Work out the finished part from the listing and answer in its coordinate system (mm). A direction names the side the tool comes from. Give positions to 0.01 mm unless a question says otherwise; leave off trailing zeros. Loops run counter-clockwise (first coordinate to the right, second up) from the corner with the lowest first, then second, coordinate; pieces in that order, holes last. Notation, with made-up numbers: M 27.5,73 L 70.5,73 A22 ccw 70.5,89 Z; hole C 10,76 d8. An arc over 180 degrees is marked long. Answer in a Markdown table with one row per item. Add a question column.
from build123d import *

# Parameters (mm, degrees)
SKETCH_1_W          = 50
SKETCH_1_H          = 15
EXTRUDE_1_DEPTH     = 18.8
SKETCH_2_W          = 46.4
SKETCH_2_H          = 15
CUT_EXTRUDE_1_DEPTH = 0.8
SKETCH_4_W          = 8.2
SKETCH_4_H          = 15
CUT_EXTRUDE_2_DEPTH = 9
SKETCH_5_W          = 8.2
SKETCH_5_H          = 1.9
CUT_EXTRUDE_3_DEPTH = 15
SKETCH_6_W          = 1.5
SKETCH_6_H          = 0.75
EXTRUDE_2_DEPTH     = 5.8
SKETCH_7_R          = 2.25
CUT_EXTRUDE_4_DEPTH = 31.004832944
CUT_EXTRUDE_START   = -30
CUT_EXTRUDE_5_DEPTH = 30


with BuildPart() as part:
    # 草图1 → 拉伸1 (new body)
    with BuildSketch(Plane(origin=(0, 0, 0), x_dir=(1, 0, 0), z_dir=(0, 1, 0))):
        Rectangle(SKETCH_1_W, SKETCH_1_H)
    extrude(amount=EXTRUDE_1_DEPTH)

    # 草图2 → 切除-拉伸1 (cut)
    with BuildSketch(Plane(origin=(0, 18.8, 0), x_dir=(-1, 0, 0), z_dir=(0, 1, 0))):
        Rectangle(SKETCH_2_W, SKETCH_2_H)
    extrude(amount=-CUT_EXTRUDE_1_DEPTH, mode=Mode.SUBTRACT)

    # 草图4 → 切除-拉伸2 (cut)
    with BuildSketch(Plane(origin=(0, 18, 0), x_dir=(-1, 0, 0), z_dir=(0, 1, 0))):
        with Locations((-19.1, 0)):
            Rectangle(SKETCH_4_W, SKETCH_4_H)
        with Locations((-9.55, 0)):
            Rectangle(SKETCH_4_W, SKETCH_4_H)
        Rectangle(SKETCH_4_W, SKETCH_4_H)
        with Locations((9.55, 0)):
            Rectangle(SKETCH_4_W, SKETCH_4_H)
        with Locations((19.1, 0)):
            Rectangle(SKETCH_4_W, SKETCH_4_H)
    extrude(amount=-CUT_EXTRUDE_2_DEPTH, mode=Mode.SUBTRACT)

    # 草图5 → 切除-拉伸3 (cut)
    with BuildSketch(Plane(origin=(0, 18, 0), x_dir=(-1, 0, 0), z_dir=(0, 1, 0))):
        with Locations((19.1, -6.55)):
            Rectangle(SKETCH_5_W, SKETCH_5_H)
        with Locations((19.1, 6.55)):
            Rectangle(SKETCH_5_W, SKETCH_5_H)
        with Locations((9.55, -6.55)):
            Rectangle(SKETCH_5_W, SKETCH_5_H)
        with Locations((9.55, 6.55)):
            Rectangle(SKETCH_5_W, SKETCH_5_H)
        with Locations((0, -6.55)):
            Rectangle(SKETCH_5_W, SKETCH_5_H)
        with Locations((0, 6.55)):
            Rectangle(SKETCH_5_W, SKETCH_5_H)
        with Locations((-9.55, -6.55)):
            Rectangle(SKETCH_5_W, SKETCH_5_H)
        with Locations((-9.55, 6.55)):
            Rectangle(SKETCH_5_W, SKETCH_5_H)
        with Locations((-19.1, -6.55)):
            Rectangle(SKETCH_5_W, SKETCH_5_H)
        with Locations((-19.1, 6.55)):
            Rectangle(SKETCH_5_W, SKETCH_5_H)
    extrude(amount=-CUT_EXTRUDE_3_DEPTH, mode=Mode.SUBTRACT)

    # 草图6 → 拉伸2 (add)
    with BuildSketch(Plane.XZ):
        Rectangle(SKETCH_6_W, SKETCH_6_H)
        with Locations((9.55, 0)):
            Rectangle(SKETCH_6_W, SKETCH_6_H)
        with Locations((-9.55, 0)):
            Rectangle(SKETCH_6_W, SKETCH_6_H)
    extrude(amount=EXTRUDE_2_DEPTH)

    # 草图7 → 切除-拉伸4 (cut, through all)
    with BuildSketch(Plane(origin=(0, 9, 0), x_dir=(-1, 0, 0), z_dir=(0, 1, 0))):
        with Locations(Location((-19.1, 0, 0), (0, 0, 90))):
            Circle(SKETCH_7_R)
        with Locations(Location((19.1, 0, 0), (0, 0, 270))):
            Circle(SKETCH_7_R)
    extrude(amount=-CUT_EXTRUDE_4_DEPTH, mode=Mode.SUBTRACT)

    # 草图8 → 切除-拉伸5 (cut)
    with BuildSketch(Plane(origin=(15, 0, 0), x_dir=(0, 0, -1), z_dir=(1, 0, 0)).offset(CUT_EXTRUDE_START)):
        Polygon((7.5, 16.8), (5.4, 14.5), (7.5, 12.3), align=None)
        Polygon((-7.5, 16.8), (-7.5, 12.3), (-5.4, 14.5), align=None)
    extrude(amount=CUT_EXTRUDE_5_DEPTH, mode=Mode.SUBTRACT)


solid = part.part
(1) Each of these flat-tipped pins is pushed along its axis until it touches: P1, Ø0.6, axis at y = -4, z = 0, coming from the -X side; P2, Ø1.2, axis at x = -9.5, y = -3, coming from the +Z side (3 decimals); P3, Ø4, axis at x = -5, z = 5, coming from the +Y side. Where does it stop, or does it pass through?
(2) The mould has two halves that part along Y. Classify faces 6 (the face through (-4.784, 13.385, 6.465)), 7 (the face through (-14, 18, 0)), 8 (the face through (-9, 6, -5.6)): pulls with the +Y half, pulls with the -Y half, needs draft (parallel to the pull), parting line crosses it, or undercut.
(3) Section D-D, the plane z = -3 is taken. Determine the outline of the cut face in (x, y), and give its area (3 significant figures).
(4) Section B-B, the plane z = 1.5 is taken. State how many separate pieces and enclosed holes the cut face has, and give its area (3 significant figures).
(5) Section A-A, the plane x = -19.1 is taken. Determine the outline of the cut face in (y, z), and give its area (3 significant figures).
(6) Section C-C, the plane y = 15.5 is taken. Determine the outline of the cut face in (x, z), and give its area (3 significant figures).
(7) Which of the six approach directions +Z, -Z, +X, -X, +Y, -Y give full straight-line access (tool end or side, diameter ignored) to faces 1 (the face through (10, 3, 7)), 2 (the face through (-19, 6, -5.6)), 3 (the face through (10, 9, 0)), 4 (the face through (-14.334, 15.666, -6.465)), 5 (the face through (-4.784, 15.634, 6.435))?
(8) Consider line 1 along X through (y, z) = (7, 0); line 2 along X through (y, z) = (17, -1.25); line 3 along Z through (x, y) = (-10, 6.75). Determine where each line is inside the solid, lowest interval first. Write a range as from..to.
Numbers:
| question | item | result |
|---|---|---|
| 1 | P1 | stops at x = -10.3 |
| 1 | P2 | stops at z = 0.375 |
| 1 | P3 | stops at y = 18 |
| 2 | face 6 | undercut |
| 2 | face 7 | pulls with the +Y half |
| 2 | face 8 | needs draft |
| 3 | outline | M -25,0 L 25,0 L 25,18.8 L 23.2,18.8 L 23.2,9 L 15,9 L 15,18 L 13.65,18 L 13.65,9 L 5.45,9 L 5.45,18 L 4.1,18 L 4.1,9 L -4.1,9 L -4.1,18 L -5.45,18 L -5.45,9 L -13.65,9 L -13.65,18 L -15,18 L -15,9 L -23.2,9 L -23.2,18.8 L -25,18.8 Z |
| 3 | area | 534 mm² |
| 4 | separate pieces | 3 |
| 4 | enclosed holes | 0 |
| 4 | area | 474 mm² |
| 5 | outline | M 0,-7.5 L 3,-7.5 L 3,-5.6 L 9,-5.6 L 9,-2.25 L 0,-2.25 Z; M 0,2.25 L 9,2.25 L 9,5.6 L 3,5.6 L 3,7.5 L 0,7.5 Z |
| 5 | area | 71.7 mm² |
| 6 | outline | M -25,-7.5 L -23.2,-7.5 L -23.2,7.5 L -25,7.5 Z; M -15,-6.31 L -13.65,-6.31 L -13.65,6.31 L -15,6.31 Z; M -5.45,-6.31 L -4.1,-6.31 L -4.1,6.31 L -5.45,6.31 Z; M 4.1,-6.31 L 5.45,-6.31 L 5.45,6.31 L 4.1,6.31 Z; M 13.65,-6.31 L 15,-6.31 L 15,6.31 L 13.65,6.31 Z; M 23.2,-7.5 L 25,-7.5 L 25,7.5 L 23.2,7.5 Z |
| 6 | area | 122 mm² |
| 7 | face 1 | +Z, +Y |
| 7 | face 2 | -Z, +Y |
| 7 | face 3 | +Z, -Z, +Y |
| 7 | face 4 | -Z |
| 7 | face 5 | +Z |
| 8 | line 1 | x = -25..-21.35, -16.85..16.85, 21.35..25 |
| 8 | line 2 | x = -25..-23.2, -15..-13.65, -5.45..-4.1, 4.1..5.45, 13.65..15, 23.2..25 |
| 8 | line 3 | z = -5.6..5.6 |
